Can you work these out from the model? Positions are in its coordinate system, mm. Face numbers are marked on the shaded views. A direction names the side the tool comes from. Give positions to 0.01 mm unless a question says otherwise; leave off trailing zeros. Write each loop counter-clockwise with the first axis right and the second up, starting at its lowest first coordinate (ties: lowest second). Pieces come first, ordered by that corner, then holes. Notation, with made-up numbers: (77, -28.5) -> (107, -28.5) arc R16 cw to (107, -23.5) -> close; hole circle Ø7 at (37.5, -26.5). An arc over 180 degrees is marked (long way). Answer as CSV lines item,"result". Start each with the question number.
1. I need wall thicknesses on line 1 (X direction, y = 3, z = 9.75); line 2 (X direction, y = -9.5, z = 8.5); line 3 (X direction, y = -1, z = 7.25). Which ranges of each line are inside material? Lowest first, please. Write a range as [from, to].
2. If we section it at B-B on x = 14: Write out the boundary of the cut face in (y, z).
3. On a 3-axis mill with a long thin cutter (end or side, diameter ignored), from which of +Z, -Z, +X, -X, +Y, -Y can I reach the whole of each face in a straight line? I mean the marked faces 3, 4 and 5. Say none if no direction works.
4. If we mould it in two halves opening along X, with no side actions, what happens to the marked faces 1 and 2? For each: pulls with the +X half, pulls with the -X half, needs draft (parallel to the pull), parting line crosses it, or undercut.
5. If we section it at A-A on z = 3.25: Count the separate pieces of the cut face and the enclosed holes in it, plus the area to 3 significant figures.
6. I'm going to push flat-ended pins straight in: P1, Ø5, axis at y = -3, z = 11.5, coming from the +X side (3 decimals); P2, Ø2.5, axis at x = -31.16, y = 0, coming from the +Z side; P3, Ø8, axis at x = 0, z = 9.5, coming from the -Y side; P4, Ø1.6, axis at x = -5, y = 4.5, coming from the +Z side. Where does each tip first touch, or does it pass through?
```python
from build123d import *

# Parameters (mm, degrees)
F1_DEPTH = 5
F0_R     = 2.25
F0_W     = 44
F0_H     = 40
F0_R_2   = 1.6
F0_R_3   = 12
F0_R_4   = 4
F2_DEPTH = 15
F3_SIZE2 = 10
F3_SIZE  = 17.5
F4_SIZE2 = 10
F4_SIZE  = 17.5


with BuildPart() as f1:
    # F0 (on Top) → F1 (new body)
    with BuildSketch(Plane.XY):
        with BuildLine():
            Line((4.8406173328, -2.5), (-12.5600405904, -2.5))
            ThreePointArc((-12.5600405904, -2.5), (-15.4689669073, -6.4807406984), (-20.1593826672, -8))
            Line((-20.1593826672, -8), (4.8406173328, -8))
            Line((4.8406173328, -8), (4.8406173328, -2.5))
        make_face()
    extrude(amount=F1_DEPTH)



with BuildPart() as f1b:
    # F0 (on Top) → F1, piece 2 (new body)
    with BuildSketch(Plane.XY):
        with BuildLine():
            ThreePointArc((-20.1593826672, 8), (-15.4689669073, 6.4807406984), (-12.5600405904, 2.5))
            Line((-12.5600405904, 2.5), (4.8406173328, 2.5))
            Line((4.8406173328, 2.5), (4.8406173328, 8))
            Line((4.8406173328, 8), (-20.1593826672, 8))
        make_face()
    extrude(amount=F1_DEPTH)


with BuildPart() as f1c:
    # F0 (on Top) → F1, piece 3 (new body)
    with BuildSketch(Plane.XY):
        with BuildLine():
            ThreePointArc((-20.1593826672, -8), (-28.1593826672, 0), (-20.1593826672, 8))
            Line((-20.1593826672, 8), (-32.1593826672, 8))
            ThreePointArc((-32.1593826672, 8), (-34.2807030107, 7.1213203436), (-35.1593826672, 5))
            Line((-35.1593826672, 5), (-35.1593826672, -5))
            ThreePointArc((-35.1593826672, -5), (-34.2807030107, -7.1213203436), (-32.1593826672, -8))
            Line((-32.1593826672, -8), (-20.1593826672, -8))
        make_face()
        with Locations((-31.1593826672, 0)):
            Circle(F0_R, mode=Mode.SUBTRACT)
    extrude(amount=F1_DEPTH)


with BuildPart() as f1d:
    # F0 (on Top) → F1, piece 4 (new body)
    with BuildSketch(Plane.XY):
        with BuildLine():
            Line((91.8406173328, 8), (79.8406173328, 8))
            ThreePointArc((79.8406173328, 8), (85.4974715823, 5.6568542495), (87.8406173328, 0))
            ThreePointArc((87.8406173328, 0), (85.4974715823, -5.6568542495), (79.8406173328, -8))
            Line((79.8406173328, -8), (91.8406173328, -8))
            ThreePointArc((91.8406173328, -8), (93.9619376764, -7.1213203436), (94.8406173328, -5))
            Line((94.8406173328, -5), (94.8406173328, 5))
            ThreePointArc((94.8406173328, 5), (93.9619376764, 7.1213203436), (91.8406173328, 8))
        make_face()
        with Locations((90.8406173328, 0)):
            Circle(F0_R, mode=Mode.SUBTRACT)
    extrude(amount=F1_DEPTH)


with BuildPart() as f1e:
    # F0 (on Top) → F1, piece 5 (new body)
    with BuildSketch(Plane.XY):
        with BuildLine():
            Line((54.8406173328, -2.5), (54.8406173328, -8))
            Line((54.8406173328, -8), (79.8406173328, -8))
            ThreePointArc((79.8406173328, -8), (75.150201573, -6.4807406984), (72.2412752561, -2.5))
            Line((72.2412752561, -2.5), (54.8406173328, -2.5))
        make_face()
    extrude(amount=F1_DEPTH)


with BuildPart() as f1f:
    # F0 (on Top) → F1, piece 6 (new body)
    with BuildSketch(Plane.XY):
        with BuildLine():
            Line((79.8406173328, 8), (54.8406173328, 8))
            Line((54.8406173328, 8), (54.8406173328, 2.5))
            Line((54.8406173328, 2.5), (72.2412752561, 2.5))
            ThreePointArc((72.2412752561, 2.5), (75.150201573, 6.4807406984), (79.8406173328, 8))
        make_face()
    extrude(amount=F1_DEPTH)


with BuildPart() as f1g:
    # F0 (on Top) → F1, piece 7 (new body)
    with BuildSketch(Plane.XY):
        with Locations((29.8406173328, 0)):
            Rectangle(F0_W, F0_H)
        with Locations((13.8406173328, -16)):
            Circle(F0_R_2, mode=Mode.SUBTRACT)
        with Locations((45.8406173328, -16)):
            Circle(F0_R_2, mode=Mode.SUBTRACT)
        with Locations((13.8406173328, 16)):
            Circle(F0_R_2, mode=Mode.SUBTRACT)
        with Locations((29.8406173328, 0)):
            Circle(F0_R_3, mode=Mode.SUBTRACT)
        with Locations((45.8406173328, 16)):
            Circle(F0_R_2, mode=Mode.SUBTRACT)
    extrude(amount=F1_DEPTH)


with BuildPart() as f1_1:
    add(f1.part)

    add(f1b.part)  # F2 merges F1b

    add(f1c.part)  # F2 merges F1c

    add(f1d.part)  # F2 merges F1d

    add(f1e.part)  # F2 merges F1e

    add(f1f.part)  # F2 merges F1f

    add(f1g.part)  # F2 merges F1g
    # F0 (on Top) → F2 (join)
    with BuildSketch(Plane.XY):
        with BuildLine():
            ThreePointArc((-12.5600405904, -2.5), (-12.2601821818, -1.2659509046), (-12.1593826672, 0))
            ThreePointArc((-12.1593826672, 0), (-12.2601821818, 1.2659509046), (-12.5600405904, 2.5))
            ThreePointArc((-12.5600405904, 2.5), (-15.4689669073, 6.4807406984), (-20.1593826672, 8))
            ThreePointArc((-20.1593826672, 8), (-28.1593826672, 0), (-20.1593826672, -8))
            ThreePointArc((-20.1593826672, -8), (-15.4689669073, -6.4807406984), (-12.5600405904, -2.5))
        make_face()
        with Locations((-20.1593826672, 0)):
            Circle(F0_R_4, mode=Mode.SUBTRACT)
        with BuildLine():
            ThreePointArc((87.8406173328, 0), (85.4974715823, 5.6568542495), (79.8406173328, 8))
            ThreePointArc((79.8406173328, 8), (75.150201573, 6.4807406984), (72.2412752561, 2.5))
            ThreePointArc((72.2412752561, 2.5), (71.8406173328, 0), (72.2412752561, -2.5))
            ThreePointArc((72.2412752561, -2.5), (75.150201573, -6.4807406984), (79.8406173328, -8))
            ThreePointArc((79.8406173328, -8), (85.4974715823, -5.6568542495), (87.8406173328, 0))
        make_face()
        with Locations((79.8406173328, 0)):
            Circle(F0_R_4, mode=Mode.SUBTRACT)
        with BuildLine():
            ThreePointArc((-12.5600405904, 2.5), (-12.2601821818, 1.2659509046), (-12.1593826672, 0))
            ThreePointArc((-12.1593826672, 0), (-12.2601821818, -1.2659509046), (-12.5600405904, -2.5))
            Line((-12.5600405904, -2.5), (4.8406173328, -2.5))
            Line((4.8406173328, -2.5), (4.8406173328, -8))
            Line((4.8406173328, -8), (4.8406173328, -20))
            Line((4.8406173328, -20), (7.8406173328, -20))
            Line((7.8406173328, -20), (7.8406173328, 20))
            Line((7.8406173328, 20), (4.8406173328, 20))
            Line((4.8406173328, 20), (4.8406173328, 8))
            Line((4.8406173328, 8), (4.8406173328, 2.5))
            Line((4.8406173328, 2.5), (-12.5600405904, 2.5))
        make_face()
        with BuildLine():
            Line((54.8406173328, 20), (51.8406173328, 20))
            Line((51.8406173328, 20), (51.8406173328, -20))
            Line((51.8406173328, -20), (54.8406173328, -20))
            Line((54.8406173328, -20), (54.8406173328, -8))
            Line((54.8406173328, -8), (54.8406173328, -2.5))
            Line((54.8406173328, -2.5), (72.2412752561, -2.5))
            ThreePointArc((72.2412752561, -2.5), (71.8406173328, 0), (72.2412752561, 2.5))
            Line((72.2412752561, 2.5), (54.8406173328, 2.5))
            Line((54.8406173328, 2.5), (54.8406173328, 8))
            Line((54.8406173328, 8), (54.8406173328, 20))
        make_face()
    extrude(amount=F2_DEPTH)

    # F3
    f3_edges = [f1_1.edges().sort_by_distance(p)[0] for p in [
        (6.340617, -20, 15),
        (6.340617, 20, 15),
    ]]
    f3_side = f1_1.faces().sort_by_distance((-7.289097, 0, 15))[0]
    chamfer(f3_edges, length=F3_SIZE, length2=F3_SIZE2, reference=f3_side)

    # F4
    f4_edges = [f1_1.edges().sort_by_distance(p)[0] for p in [
        (53.340617, -20, 15),
        (53.340617, 20, 15),
    ]]
    f4_side = f1_1.faces().sort_by_distance((66.970331, 0, 15))[0]
    chamfer(f4_edges, length=F4_SIZE, length2=F4_SIZE2, reference=f4_side)


solid = f1_1.part
```
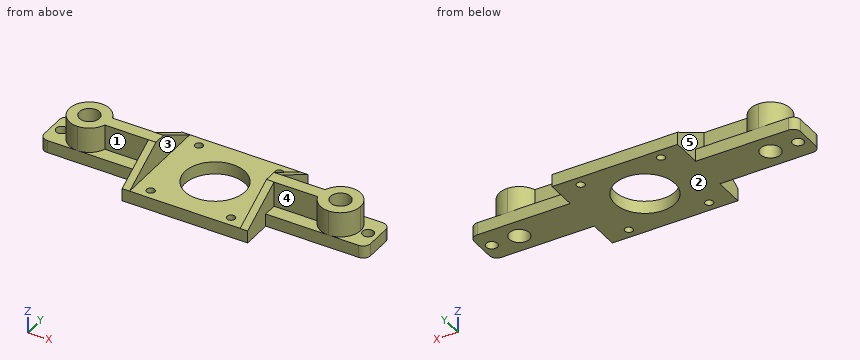
Computed values:
1,line 1,"x = [-27.58, -22.81], [-17.51, -12.74], [4.84, 7.84], [51.84, 54.84], [72.42, 77.19], [82.49, 87.26]"
1,line 2,"x = [4.84, 7.84], [51.84, 54.84]"
1,line 3,"x = [-28.1, -24.03], [-16.29, 7.84], [51.84, 75.97], [83.71, 87.78]"
2,outline,"(-20, 0) -> (-17.59, 0) -> (-17.59, 5) -> (-20, 5) -> close; (-14.41, 0) -> (14.41, 0) -> (14.41, 5) -> (-14.41, 5) -> close; (17.59, 0) -> (20, 0) -> (20, 5) -> (17.59, 5) -> close"
3,face 3,"+Z, +Y, -Y"
3,face 4,"+Z, -Y"
3,face 5,"+Z, +Y"
4,face 1,"undercut"
4,face 2,"needs draft"
5,separate pieces,"1"
5,enclosed holes,"9"
5,area,"2,660 mm2"
6,P1,"stops at x = 87.825"
6,P2,"passes through"
6,P3,"stops at y = -2.5"
6,P4,"stops at z = 5"
